Could you check a few things on this model? Use its own coordinates, in mm. Face numbers are marked on the shaded views. A direction names the side the tool comes from. Give positions to 0.01 mm unless a question says otherwise; leave off trailing zeros. Loops run counter-clockwise (first coordinate to the right, second up) from the corner with the lowest first, then second, coordinate; pieces in that order, holes last. Notation, with made-up numbers: M -14.5,50.5 L -2.5,50.5 A19 cw -2.5,75.5 Z; hole C -35.75,0 d10. An arc over 180 degrees is marked long. Answer in a Markdown table with one row per item. Add a question column.
1. Thinking about a two-plate mould opening in Y: for the marked faces 1, 2 and 3, which applies, released by +Y, released by -Y, zero draft, split by the parting line, or undercut?
2. Which directions (+Z, -Z, +X, -X, +Y, -Y) give clear straight access to the entire face, cutting with the end or side of a thin tool? Please do the marked faces 4 and 5.
3. I need wall thicknesses on line 1 along Z through (x, y) = (-0.5, -0.5); line 2 along Y through (x, z) = (-0.25, 3); line 3 along Y through (x, z) = (-1, -0.25). Which ranges of each line are inside material? Lowest first, please. Write a range as from..to.
4. I'm going to push a flat-ended pin straight in: pin 1 Ø3 at (x, z) = (-2, -2) entering from +Y. Where does the tip first touch, or does it pass through?
5. If we section it at B-B on z = -0.5: List the corners of the cut face in (x, y) for me.
6. If we section it at A-A on x = 0: List the corners of the cut face in (y, z) for me.
```python
from build123d import *

# Parameters (mm, degrees)
CUT_EXTRUDE_1_DEPTH = 1.5
FILLET_1_R          = 0.3


with BuildPart() as part:
    # 草图1 → 旋转1 (revolve)
    with BuildSketch(Plane(origin=(0, 0, 0), x_dir=(0, 0, -1), z_dir=(1, 0, 0))):
        Polygon((-4, 0), (-4, 3), (-3.1, 3), (-1.6, 1.5), (3.7, 1.5), (4, 1.2), (4, 0), align=None)
    revolve(axis=Axis((0, 0, -4), (0, 0, 1)))

    # 草图2 → 切除-拉伸1 (cut)
    with BuildSketch(Plane.XY.offset(4)):
        Polygon((1.154700538, 0), (0.577350269, 1), (-0.577350269, 1), (-1.154700538, 0), (-0.577350269, -1), (0.577350269, -1), align=None)
    extrude(amount=-CUT_EXTRUDE_1_DEPTH, mode=Mode.SUBTRACT)

    # 圆角1
    fillet_1_edges = [part.edges().sort_by_distance(p)[0] for p in [
        (0, -3, 4),
    ]]
    fillet(fillet_1_edges, radius=FILLET_1_R)


solid = part.part
```
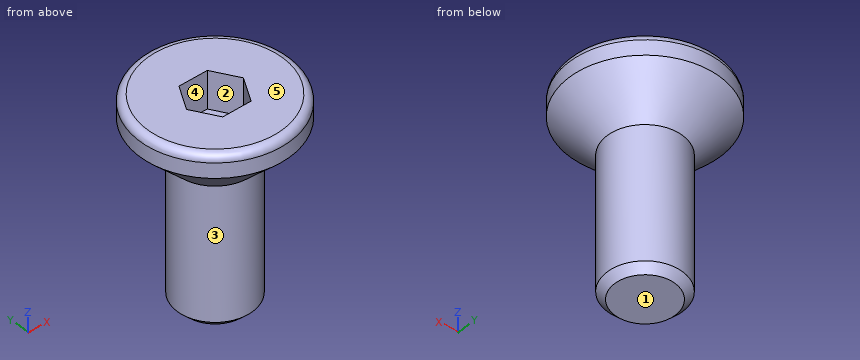
Results:
| question | item | result |
|---|---|---|
| 1 | face 1 | zero draft |
| 1 | face 2 | undercut |
| 1 | face 3 | split by the parting line |
| 2 | face 4 | +Z |
| 2 | face 5 | +Z, +X, -X, +Y, -Y |
| 3 | line 1 | -4..2.5 |
| 3 | line 2 | -2.89..-1, 1..2.89 |
| 3 | line 3 | -1.12..1.12 |
| 4 | pin 1 | y = 1.41 |
| 5 | outline | C 0,0 d3 |
| 6 | outline | M -3,3.1 L -1.5,1.6 L -1.5,-3.7 L -1.2,-4 L 1.2,-4 L 1.5,-3.7 L 1.5,1.6 L 3,3.1 L 3,3.7 A0.3 ccw 2.7,4 L 1,4 L 1,2.5 L -1,2.5 L -1,4 L -2.7,4 A0.3 ccw -3,3.7 Z |
